Answer from the drawing. Dimensions are ordinates in mm from the lowest x, y and z of the part. A direction names the side the tool comes from. Give positions to 0.01 mm unless a question says otherwise; leave off trailing zeros. Write each loop counter-clockwise with the first axis right and the second up, starting at its lowest first coordinate (ties: lowest second). Pieces come first, ordered by that corner, then holes.
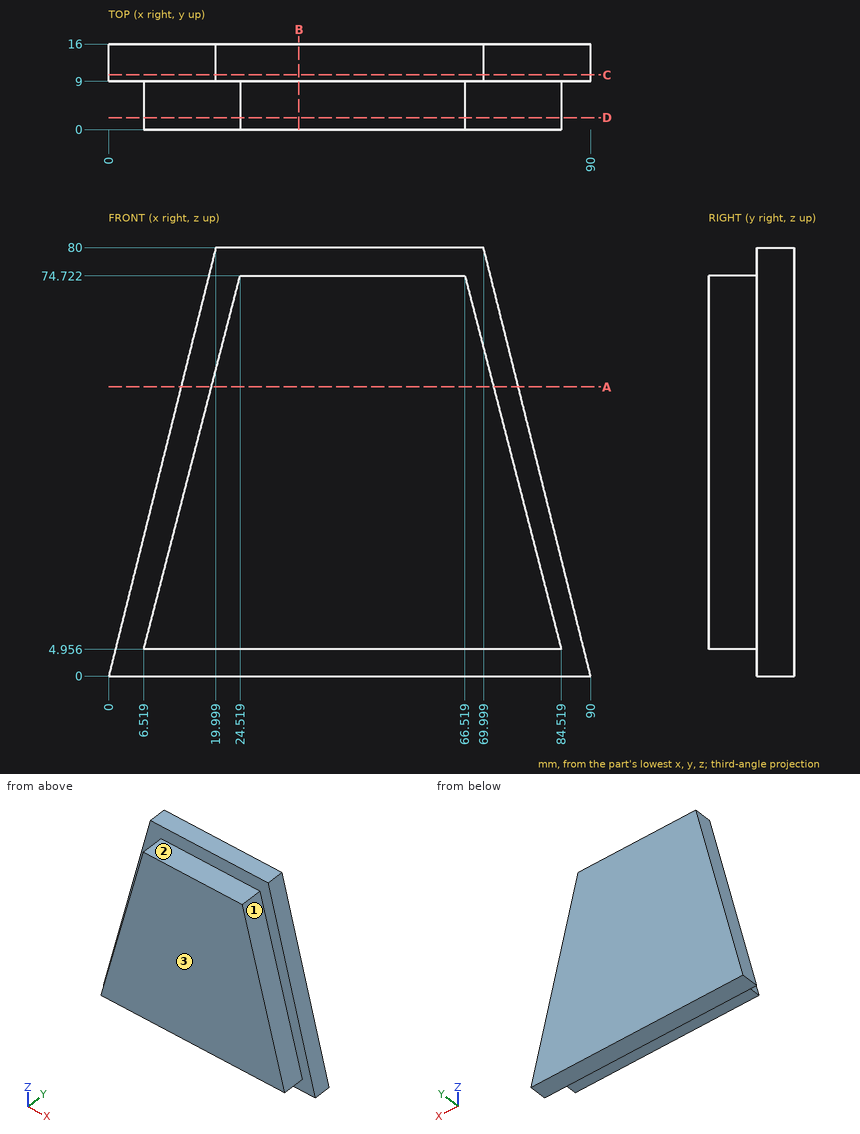
Item 1: A cutting plane is placed at C-C, the plane y = 10.25. Give the vertices of the cut face in (x, z).
Conclusion:
outline: (0, 0) - (90, 0) - (70, 80) - (20, 80) - close
Item 2: Consider probe 1 along Z at (x, y) = (65.5, 2.75) (1 decimal); probe 2 along Y at (x, z) = (82, 16); probe 3 along X at (y, z) = (7, 37). Determine where each line is inside the solid, lowest interval first.
Conclusion:
probe 1: z = 5 to 74.7
probe 2: y = 9 to 16
probe 3: x = 14.79 to 76.25
Item 3: A cutting plane is placed at B-B, the plane x = 35.5. Give the vertices of the cut face in (y, z) (1 decimal).
Conclusion:
outline: (0, 5) - (9, 5) - (9, 0) - (16, 0) - (16, 80) - (9, 80) - (9, 74.7) - (0, 74.7) - close
Item 4: A cutting plane is placed at A-A, the plane z = 54. Give the vertices of the cut face in (x, y) (1 decimal).
Conclusion:
outline: (13.5, 9) - (19.2, 9) - (19.2, 0) - (71.9, 0) - (71.9, 9) - (76.5, 9) - (76.5, 16) - (13.5, 16) - close
Item 5: Each of these flat-tipped pins is pushed along its axis until it touches: P1, Ø1, axis at y = 11, z = 38.5, coming from the -X side; P2, Ø6, axis at y = 5, z = 14.5, coming from the -X side; P3, Ø2.5, axis at x = 42.5, y = 3, coming from the +Z side. Where does it stop, or does it pass through?
Conclusion:
P1: stops at x = 9.5
P2: stops at x = 8.21
P3: stops at z = 74.72
Item 6: Which of the six approach directions +Z, -Z, +X, -X, +Y, -Y give full straight-line access (tool end or side, diameter ignored) to the marked faces 1, 2 and 3?
Conclusion:
face 1: +Z, +X, -Y
face 2: +Z, +X, -X, -Y
face 3: +Z, -Z, +X, -X, -Y
Item 7: A cutting plane is placed at D-D, the plane y = 2.25. Give the vertices of the cut face in (x, z) (1 decimal).
Conclusion:
outline: (6.5, 5) - (84.5, 5) - (66.5, 74.7) - (24.5, 74.7) - close
